```python
from build123d import *

# Parameters (mm, degrees)
F0_W     = 268
F0_H     = 168
F1_DEPTH = 2
F3_DEPTH = 268
F6_DEPTH = 168
F7_DEPTH = 268
F8_W     = 10
F8_H     = 22.5
F9_DEPTH = 25


with BuildPart() as f1:
    # F0 (on Top) → F1 (new body)
    with BuildSketch(Plane.XY):
        with Locations((134, -84)):
            Rectangle(F0_W, F0_H)
    extrude(amount=F1_DEPTH)

    # F2 (on face) → F3 (join)
    with BuildSketch(Plane.YZ.offset(268)):
        with BuildLine():
            Line((-168, 2), (-170, 2))
            ThreePointArc((-170, 2), (-169.414214, 0.585786), (-168, 0))
            Line((-168, 0), (-168, 2))
        make_face()
    extrude(amount=-F3_DEPTH)

    # F4 (on face) → F6 (join)
    with BuildSketch(Plane(origin=(0, 0, 0), x_dir=(-1, 0, 0), z_dir=(0, 1, 0))):
        with BuildLine():
            Line((0, 2), (0, 0))
            ThreePointArc((0, 0), (1.414214, 0.585786), (2, 2))
            Line((2, 2), (0, 2))
        make_face()
        with BuildLine():
            Line((-268, 2), (-270, 2))
            ThreePointArc((-270, 2), (-269.414214, 0.585786), (-268, 0))
            Line((-268, 0), (-268, 2))
        make_face()
    extrude(amount=-F6_DEPTH)

    # F5 (on face) → F7 (join)
    with BuildSketch(Plane.YZ.offset(268)):
        with BuildLine():
            Line((0, 2), (0, 0))
            ThreePointArc((0, 0), (1.414214, 0.585786), (2, 2))
            Line((2, 2), (0, 2))
        make_face()
    extrude(amount=-F7_DEPTH)

    # F8 (on face) → F9 (cut)
    with BuildSketch(Plane.XY.offset(2)):
        with Locations((263, -39.25)):
            Rectangle(F8_W, F8_H)
        with Locations((263, -126.75)):
            Rectangle(F8_W, F8_H)
        with Locations((5, -126.75)):
            Rectangle(F8_W, F8_H)
        with Locations((5, -39.25)):
            Rectangle(F8_W, F8_H)
    extrude(amount=-F9_DEPTH, mode=Mode.SUBTRACT)


solid = f1.part
```
Input: part model. Units: mm. Frame: model coordinates. Coordinates: 2 decimals unless noted, no trailing zeros. Write each loop counter-clockwise with the first axis right and the second up, starting at its lowest first coordinate (ties: lowest second). Pieces come first, ordered by that corner, then holes. Notation, with made-up numbers: M -7.75,83 L 29.25,83 A17 cw 29.25,111 Z; hole C 30.5,84.25 d3. An arc over 180 degrees is marked long. Use one line per item in the form item = value.
Q1. Section B-B (z = 0.6). Return loops of the section in (x, y).
Answer below:
outline = M -1.43,-168 L 0,-168 L 0,-169.43 L 268,-169.43 L 268,-168 L 269.43,-168 L 269.43,0 L 268,0 L 268,1.43 L 0,1.43 L 0,0 L -1.43,0 Z; hole M 0,-138 L 10,-138 L 10,-115.5 L 0,-115.5 Z; hole M 0,-50.5 L 10,-50.5 L 10,-28 L 0,-28 Z; hole M 258,-138 L 268,-138 L 268,-115.5 L 258,-115.5 Z; hole M 258,-50.5 L 268,-50.5 L 268,-28 L 258,-28 Z
Q2. First-contact query: pin 1 (0.6 mm diameter, centred on x = 264.5, z = 0.5, fed in from -Y); pin 2 (0.6 mm diameter, centred on y = -168.5, z = 0.5, fed in from +X); pin 3 (1 mm diameter, centred on y = -126, z = 1, fed in from -X). Flat tips, straight axial feed; report the tip coordinate or a pass-through.
Answer below:
pin_1 = -169.6
pin_2 = 268
pin_3 = -1.94
Q3. Material intervals for probe 1 along X at (y, z) = (-39, 1.8); probe 2 along X at (y, z) = (-125, 1.4); probe 3 along Y at (x, z) = (215, 1.7), sorted ascending. Write a range as from..to.
Answer below:
probe_1 = -1.99..0, 10..258, 268..269.99
probe_2 = -1.91..0, 10..258, 268..269.91
probe_3 = -169.98..1.98
Q4. Section A-A (y = -131). Return loops of the section in (x, z), plus the area to 3 significant figures.
Answer below:
outline = M -2,2 A2 ccw 0,0 L 0,2 Z; M 10,0 L 258,0 L 258,2 L 10,2 Z; M 268,0 A2 ccw 270,2 L 268,2 Z
area = 502 mm²
